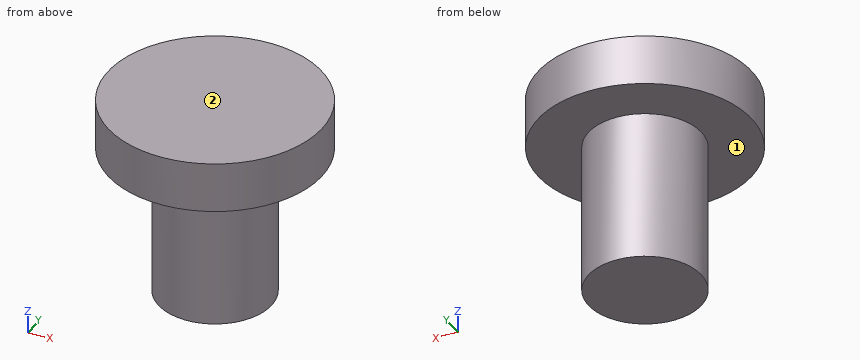
Autodesk Inventor part; units mm, degrees
ref_plane "YZ Plane" through (0, 0, 0) normal (1, 0, 0) x (0, 1, 0)
ref_plane "XZ Plane" through (0, 0, 0) normal (0, 1, 0) x (-1, 0, 0)
ref_plane "XY Plane" through (0, 0, 0) normal (0, 0, 1) x (1, 0, 0)
sketch "Sketch1" plane through (0, 0, 0) normal (0, 0, 1) x (1, 0, 0)
  circle A0 centre (0, 0) radius 4.25
  dimension "d0" = 8.5
extrude "Extrusion1" add sketch "Sketch1" along normal blind 2
sketch "Sketch2" plane through (0, 0, 0) normal (0, 0, -1) x (-1, 0, 0)
  circle A0 centre (0, 0) radius 2.25
  dimension "d3" = 4.5
extrude "Extrusion2" add sketch "Sketch2" along normal blind 6
sketch "Sketch3" plane through (0, 0, 2) normal (0, 0, 1) x (1, 0, 0)
  circle A0 centre (0, 0) radius 2.25
  circle A1 centre (0, 0) radius 4.25
  line L0 (-4.25, 0) -> (-2.125, 3.6806)
  line L1 (-2.125, 3.6806) -> (2.125, 3.6806)
  line L2 (2.125, 3.6806) -> (4.25, 0)
  line L3 (4.25, 0) -> (2.125, -3.6806)
  line L4 (2.125, -3.6806) -> (-2.125, -3.6806)
  line L5 (-2.125, -3.6806) -> (-4.25, 0)
extrude "Extrusion3" add sketch "Sketch3" against normal blind 2 contours L2 A1 | A1 L3 | L1 A1 | A1 L4 | L0 A1 | A1 L5
thread "Thread2"
properties part number "vida"
Read the model definition and answer for the solid it produces. Units are mm, in the model's axes. Face numbers are marked on the shaded views. A direction names the side the tool comes from. Coordinates: 2 decimals unless noted, no trailing zeros. Loops run counter-clockwise (first coordinate to the right, second up) from the corner with the lowest first, then second, coordinate; pieces in that order, holes last. Notation, with made-up numbers: (-1, 30.25) -> (53, 30.25) arc R25 ccw to (53, 51.25) -> close; hole circle Ø10 at (15.25, -40). An arc over 180 degrees is marked (long way). Return JSON: item names as keys, results as strings.
Item 1: A flat-ended cylindrical pin translates along its axis: P1, Ø1.5, axis at y = 0.5, z = -1.5, coming from the +X side. Find the tip coordinate at first contact, or state that the pin passes through.
Answers:
{"P1": "stops at x = 2.25"}
Item 2: For the marked faces 1 and 2, determine the directions among +Z, -Z, +X, -X, +Y, -Y from which every point of the face is accessible in a straight line to the end or side of a thin tool.
Answers:
{"face 1": "-Z", "face 2": "+Z, +X, -X, +Y, -Y"}
Item 3: Find section D-D (z = -4.5). Determine the outline of the cut face in (x, y).
Answers:
{"outline": "circle Ø4.5 at (0, 0)"}
Item 4: Find section C-C (z = 0.5). Determine the outline of the cut face in (x, y).
Answers:
{"outline": "circle Ø8.5 at (0, 0)"}
Item 5: Find the intervals of material crossed by probe 1 along Z at (x, y) = (1.25, -3.75); probe 2 along X at (y, z) = (-3, 1.75); probe 3 along Y at (x, z) = (2, -2.25), in increasing order.
Answers:
{"probe 1": "z = 0 to 2", "probe 2": "x = -3.01 to 3.01", "probe 3": "y = -1.03 to 1.03"}
Item 6: Find section A-A (x = 0). Determine the outline of the cut face in (y, z).
Answers:
{"outline": "(-4.25, 0) -> (-2.25, 0) -> (-2.25, -6) -> (2.25, -6) -> (2.25, 0) -> (4.25, 0) -> (4.25, 2) -> (-4.25, 2) -> close"}
